For this review, use the dimensioned drawing (mm, ordinates from the lowest corner) and the shaded views. A direction names the side the tool comes from. Coordinates: 2 decimals unless noted, no trailing zeros. Loops run counter-clockwise (first coordinate to the right, second up) from the corner with the lowest first, then second, coordinate; pieces in that order, holes last. Notation, with made-up numbers: (84, 5.25) -> (104, 5.25) arc R24 cw to (104, 42.25) -> close; hole circle Ø9 at (1.5, 23.25). An arc over 180 degrees is marked (long way). Use one line per item in the form item = value. Start each with the question number.
1. Machinability: for the marked faces 5 and 6, which of the approach directions +Z, -Z, +X, -X, +Y, -Y give a long, thin tool a straight path to every point of the face, cutting with its end or side? Answer none if there is none.
2. Consider section B-B (z = 22). State the section outline as (x, y) points.
3. Wall thickness on line 1 (X direction, y = 1.5, z = 5); line 2 (X direction, y = 27.5, z = 21.5): over which ranges is each line inside the solid? List them lowest first. Write a range as from..to.
4. The part is to be moulded in two halves that separate along X. For the marked faces 1, 2, 3 and 4, say which applies: released by +X, released by -X, zero draft, split by the parting line, or undercut.
5. Consider section A-A (x = 65). State the section outline as (y, z) points, then the cut area to 3 significant figures.
6. For pin 1 (2.5 mm diameter, centred on x = 8, y = 30, fed in from -Z); pin 2 (15 mm diameter, centred on y = 18, z = 38.5, fed in from -X); pin 3 (5 mm diameter, centred on y = 41.5, z = 15, fed in from +X); pin 4 (3 mm diameter, centred on x = 65, z = 5, fed in from +Y), all flat-tipped, find the tip position at first contact; note any pin that passes through.
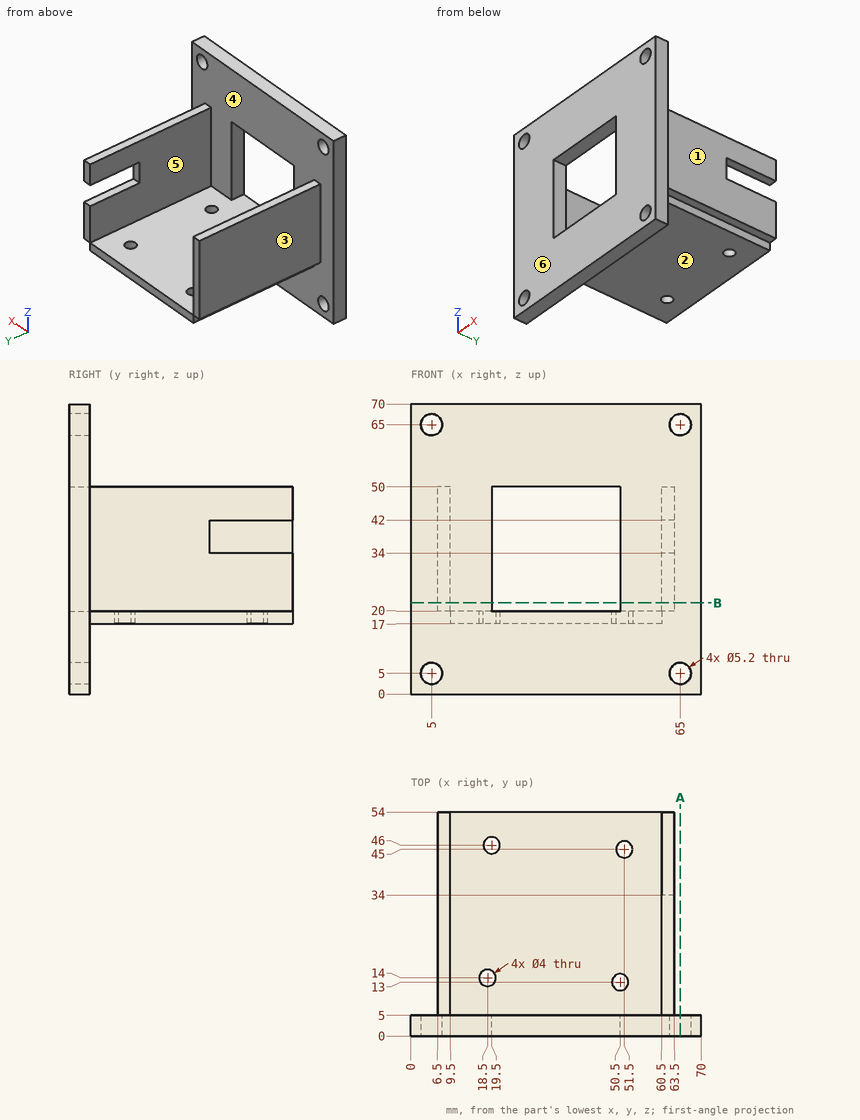
Geometry check:
q1.face_5 = +Z, +Y
q1.face_6 = +Z, -Z, +X, -X, -Y
q2.outline = (0, 0) -> (19.5, 0) -> (19.5, 5) -> (9.5, 5) -> (9.5, 54) -> (6.5, 54) -> (6.5, 5) -> (0, 5) -> close; (50.5, 0) -> (70, 0) -> (70, 5) -> (63.5, 5) -> (63.5, 54) -> (60.5, 54) -> (60.5, 5) -> (50.5, 5) -> close
q3.line_1 = 0..2.4, 7.6..62.4, 67.6..70
q3.line_2 = 6.5..9.5, 60.5..63.5
q4.face_1 = released by +X
q4.face_2 = zero draft
q4.face_3 = released by -X
q4.face_4 = undercut
q5.outline = (0, 0) -> (5, 0) -> (5, 2.4) -> (0, 2.4) -> close; (0, 7.6) -> (5, 7.6) -> (5, 62.4) -> (0, 62.4) -> close; (0, 67.6) -> (5, 67.6) -> (5, 70) -> (0, 70) -> close
q5.area = 298 mm²
q6.pin_1 = 20
q6.pin_2 = 6.5
q6.pin_3 = 60.5
q6.pin_4 = through
